```python
from build123d import *

# Parameters (mm, degrees)
F0_R     = 25.4
F0_W     = 457.2
F0_H     = 101.6
F0_R_2   = 21.43125
F1_DEPTH = 19.05
F2_DEPTH = 19.05
F3_SIZE  = 3.175


with BuildPart() as f1:
    # F0 (on Front) → F1 (new body)
    with BuildSketch(Plane.XZ):
        with BuildLine():
            ThreePointArc((228.6, 76.2), (221.160512, 94.160512), (203.2, 101.6))
            Line((203.2, 101.6), (-203.2, 101.6))
            ThreePointArc((-203.2, 101.6), (-221.160512, 94.160512), (-228.6, 76.2))
            Line((-228.6, 76.2), (-228.6, 0))
            Line((-228.6, 0), (228.6, 0))
            Line((228.6, 0), (228.6, 76.2))
        make_face()
        with Locations((-155.448, 57.15)):
            Circle(F0_R, mode=Mode.SUBTRACT)
        with Locations((155.702, 57.15)):
            Circle(F0_R, mode=Mode.SUBTRACT)
        with Locations((0, -50.8)):
            Rectangle(F0_W, F0_H)
        with Locations((-156.2735, -57.15)):
            Circle(F0_R_2, mode=Mode.SUBTRACT)
        with Locations((156.464, -57.15)):
            Circle(F0_R_2, mode=Mode.SUBTRACT)
    extrude(amount=F1_DEPTH)

    # F0 (on Front) → F2 (join)
    with BuildSketch(Plane.XZ):
        with BuildLine():
            ThreePointArc((228.6, 76.2), (221.160512, 94.160512), (203.2, 101.6))
            Line((203.2, 101.6), (-203.2, 101.6))
            ThreePointArc((-203.2, 101.6), (-221.160512, 94.160512), (-228.6, 76.2))
            Line((-228.6, 76.2), (-228.6, 0))
            Line((-228.6, 0), (228.6, 0))
            Line((228.6, 0), (228.6, 76.2))
        make_face()
        with Locations((-155.448, 57.15)):
            Circle(F0_R, mode=Mode.SUBTRACT)
        with Locations((155.702, 57.15)):
            Circle(F0_R, mode=Mode.SUBTRACT)
    extrude(amount=-F2_DEPTH)

    # F3
    f3_edges = [f1.edges().sort_by_distance(p)[0] for p in [
        (-203.2, 0, 101.6),
        (-228.6, -19.05, -12.7),
        (-228.6, 19.05, 38.1),
    ]]
    chamfer(f3_edges, length=F3_SIZE)


solid = f1.part
```
Source: CAD feature listing. Evaluate the final solid. Frame: model axes, mm. A direction names the side the tool comes from. Round coordinates to 2 decimals unless told otherwise and drop trailing zeros. Loops run counter-clockwise (first coordinate to the right, second up) from the corner with the lowest first, then second, coordinate; pieces in that order, holes last.
1. Ray query, L1, parallel to X at y = -10, z = 57; L2, parallel to Z at x = 157, y = -8; L3, parallel to Z at x = 68, y = 12. Return the intervals inside material, ascending.
2. Section query B-B on y = -5.5. Output: boundary loops of the cut face in (x, z).
3. Section query C-C on z = 57.15. Output: boundary loops of the cut face in (x, y) (3 decimals).
4. Section query A-A on z = -57.15. Output: boundary loops of the cut face in (x, y) (3 decimals).
5. Section query D-D on x = -145. Output: boundary loops of the cut face in (y, z) (3 decimals).
6. Access query for faces 1 (the flat face through (-3, 9, 0)), 2 (the flat face through (228.6, -4, 6)). Directions: +Z, -Z, +X, -X, +Y, -Y. A direction counts if a zero-diameter tool reaches every point of the face in a straight line with its end or side. Return the directions, or none.
7. Contact query for a flat-ended pin moving along its axis: pin 1 (5.5 mm diameter, centred on x = -85.5, y = 12.5, fed in from -Z). Output: stop coordinate, or through.
8. Mould query, pull axis X, two halves, no side actions, for faces 3 (the cylindrical face through (176.9, -9.4, -50.7)), 4 (the flat face through (-3, 0, -50)), 5 (the conical face through (-219.1, -18.54, 92.45)). Classes: released by +X, released by -X, zero draft, split by the parting line, or undercut.
Answers below:
1. L1: x = -228.6 to -180.85, -130.05 to 130.3, 181.1 to 228.6
1. L2: z = -101.6 to -78.57, -35.73 to 31.78, 82.52 to 101.6
1. L3: z = 0 to 101.6
2. outline: (-228.6, -101.6) - (228.6, -101.6) - (228.6, 76.2) arc R25.4 ccw to (203.2, 101.6) - (-203.2, 101.6) arc R25.4 ccw to (-228.6, 76.2) - close; hole circle Ø50.8 at (-155.45, 57.15); hole circle Ø42.86 at (-156.27, -57.15); hole circle Ø50.8 at (155.7, 57.15); hole circle Ø42.86 at (156.46, -57.15)
3. outline: (-228.6, -15.875) - (-225.425, -19.05) - (-180.848, -19.05) - (-180.848, 19.05) - (-225.425, 19.05) - (-228.6, 15.875) - close; (-130.048, -19.05) - (130.302, -19.05) - (130.302, 19.05) - (-130.048, 19.05) - close; (181.102, -19.05) - (225.425, -19.05) - (228.6, -15.875) - (228.6, 15.875) - (225.425, 19.05) - (181.102, 19.05) - close
4. outline: (-228.6, -15.875) - (-225.425, -19.05) - (-177.705, -19.05) - (-177.705, 0) - (-228.6, 0) - close; (-134.842, -19.05) - (135.033, -19.05) - (135.033, 0) - (-134.842, 0) - close; (177.895, -19.05) - (225.425, -19.05) - (228.6, -15.875) - (228.6, 0) - (177.895, 0) - close
5. outline: (-19.05, -101.6) - (0, -101.6) - (0, -75.377) - (-19.05, -75.377) - close; (-19.05, -38.923) - (0, -38.923) - (0, 0) - (19.05, 0) - (19.05, 33.998) - (-19.05, 33.998) - close; (-19.05, 80.302) - (19.05, 80.302) - (19.05, 98.425) - (15.875, 101.6) - (-15.875, 101.6) - (-19.05, 98.425) - close
6. face 1: -Z, +X, -X, +Y
6. face 2: +Z, -Z, +X, +Y, -Y
7. pin 1: stops at z = 0
8. face 3: undercut
8. face 4: zero draft
8. face 5: released by -X
